Autodesk Inventor part; units mm, degrees
ref_plane "YZ Plane" through (0, 0, 0) normal (1, 0, 0) x (0, 1, 0)
ref_plane "XZ Plane" through (0, 0, 0) normal (0, 1, 0) x (-1, 0, 0)
ref_plane "XY Plane" through (0, 0, 0) normal (0, 0, 1) x (1, 0, 0)
sketch "Skizze1" plane through (0, 0, 0) normal (0, 0, 1) x (1, 0, 0)
  line L0 (-14, 0) -> (14, 0)
  line L1 (0, -4.75) -> (0, 23.25)
  line L2 (-10, -0.75) -> (10, -0.75)
  line L3 (10, -0.75) -> (10, 0.75)
  line L4 (10, 0.75) -> (-10, 0.75)
  line L5 (-10, 0.75) -> (-10, -0.75)
  line L6 (-10, -0.75) -> (-8.5, -0.75)
  line L7 (-8.5, -0.75) -> (-8.5, 19.25)
  line L8 (-8.5, 19.25) -> (-10, 19.25)
  line L9 (-10, 19.25) -> (-10, -0.75)
  point P0 (0, 0)
  dimension "d0" = 20
  dimension "d1" = 1.5
  dimension "d2" = 1.5
  dimension "d3" = 20
extrude "Extrusion1" add sketch "Skizze1" along normal blind 55
sketch "Skizze2" plane through (-8.5, 0.75, 0) normal (0, 1, 0) x (1, 0, 0)
  line L0 (0, -55) -> (0, 0)
  line L1 (18.5, -55) -> (0, -55)
  line L2 (18.5, 0) -> (18.5, -55)
  line L3 (18.5, 0) -> (0, 0)
  circle A0 centre (9.5, -49) radius 2.5
  circle A1 centre (9.5, -6) radius 2.5
  circle A2 centre (9.5, -27.5) radius 2.5
  line L4 (18.5, -55) -> (0, -55)
  line L5 (18.5, 0) -> (0, 0)
  point P0 (8.5, 0)
  dimension "d6" = 5
  dimension "d7" = 5
  dimension "d8" = 6
  dimension "d9" = 6
  dimension "d10" = 9
  dimension "d13" = 5
  dimension "d15" = 55
  dimension "d16" = 27.5
extrude "Extrusion2" cut sketch "Skizze2" against normal blind 1.5 contours A0 | A1 | A2
sketch "Skizze3" plane through (-8.5, 0.75, 0) normal (1, 0, 0) x (0, 0, -1)
  circle A0 centre (-36, 11) radius 1.5
  line L0 (-55, 0) -> (0, 0)
  line L1 (0, 0) -> (0, 18.5)
  line L2 (0, 18.5) -> (-55, 18.5)
  line L3 (-55, 0) -> (-55, 18.5)
  circle A1 centre (-19, 11) radius 1.5
  point P0 (0, -0.75)
  dimension "d17" = 3
  dimension "d18" = 7.5
  dimension "d19" = 19
  dimension "d22" = 3
  dimension "d23" = 19
  dimension "d24" = 7.5
extrude "Extrusion3" cut sketch "Skizze3" against normal blind 1.5 contours A0 | A1
equation "\"d9\" = d8"
equation "\"d16\" = 0.5 * d15"
equation "\"d22\" = d17"
equation "\"d23\" = d19"
equation "\"d24\" = d18"
properties part number "Z-Stage_Wheel_plate_20x20" material "Aluminium 6061"
Check sheet for the modelled part. Datum: model origin and axes. Units: mm. A direction names the side the tool comes from. Coordinates: 2 decimals unless noted, no trailing zeros. Order: outer loops, then holes, each group sorted by start corner. A loop starts at its lowest first (then second) coordinate and runs counter-clockwise, first axis right, second up. Notation, with made-up numbers: (13.5, -34) -> (65.5, -34) arc R17 ccw to (65.5, -18) -> close; hole circle Ø5 at (-34.75, 12). An arc over 180 degrees is marked (long way). Write item = value, one per line. Start each with the question number.
1) Cross-section at D-D (z = 29). Enter the section's corners in (x, y).
2) Go/stop test with flat-tipped pins: P1, Ø3, axis at y = 15, z = 12.5, coming from the +X side; P2, Ø1, axis at x = 6.5, z = 38, coming from the +Y side. Record where each tip stops, or that it passes through.
3) Material ranges on L1, parallel to Z at x = 1, y = -0.2; L2, parallel to X at y = -0.05, z = 6; L3, parallel to Y at x = -9.3, z = 36, recorded low to high.
4) Cross-section at A-A (z = 36). Enter the section's corners in (x, y), then the cut area to 4 significant figures.
5) Cross-section at C-C (x = 2.75). Enter the section's corners in (y, z).
6) Access from +Z, -Z, +X, -X, +Y, -Y to the whole of each face (thin tool, end or side, straight path). Record for faces 5 (the flat face through (-3, 0.75, 27)), 6 (the cylindrical face through (-9.24, 10.84, 37.19)).
7) Mould release check, pull along Z, two halves, no side actions. Record for faces 1 (the flat face through (-8.5, 10, 27)), 2 (the cylindrical face through (2.34, 0.01, 3.89)), 3 (the cylindrical face through (-9.2, 11.8, 20.5)), 4 (the flat face through (-9, 5, 0)): +Z half, -Z half, draft (parallel to the pull), parting line (faces both ways), or undercut.
8) Cross-section at B-B (y = 11.75). Enter the section's corners in (x, z), then the cut area to 3 significant figures.
Ans:
q1.outline = (-10, -0.75) -> (-1, -0.75) -> (-1, 0.75) -> (-8.5, 0.75) -> (-8.5, 19.25) -> (-10, 19.25) -> close; (3, -0.75) -> (10, -0.75) -> (10, 0.75) -> (3, 0.75) -> close
q2.P1 = -8.5
q2.P2 = 0.75
q3.L1 = 0 to 3.5, 8.5 to 25, 30 to 46.5, 51.5 to 55
q3.L2 = -10 to -1.5, 3.5 to 10
q3.L3 = -0.75 to 10.25, 13.25 to 19.25
q4.outline = (-10, -0.75) -> (10, -0.75) -> (10, 0.75) -> (-8.5, 0.75) -> (-8.5, 10.25) -> (-10, 10.25) -> close; (-10, 13.25) -> (-8.5, 13.25) -> (-8.5, 19.25) -> (-10, 19.25) -> close
q4.area = 53.25 mm²
q5.outline = (-0.75, 0) -> (0.75, 0) -> (0.75, 4.21) -> (-0.75, 4.21) -> close; (-0.75, 7.79) -> (0.75, 7.79) -> (0.75, 25.71) -> (-0.75, 25.71) -> close; (-0.75, 29.29) -> (0.75, 29.29) -> (0.75, 47.21) -> (-0.75, 47.21) -> close; (-0.75, 50.79) -> (0.75, 50.79) -> (0.75, 55) -> (-0.75, 55) -> close
q6.face_5 = +Z, -Z, +X, +Y
q6.face_6 = +X, -X
q7.face_1 = draft
q7.face_2 = undercut
q7.face_3 = undercut
q7.face_4 = -Z half
q8.outline = (-10, 0) -> (-8.5, 0) -> (-8.5, 17.5) -> (-10, 17.5) -> close; (-10, 20.5) -> (-8.5, 20.5) -> (-8.5, 34.5) -> (-10, 34.5) -> close; (-10, 37.5) -> (-8.5, 37.5) -> (-8.5, 55) -> (-10, 55) -> close
q8.area = 73.5 mm²
